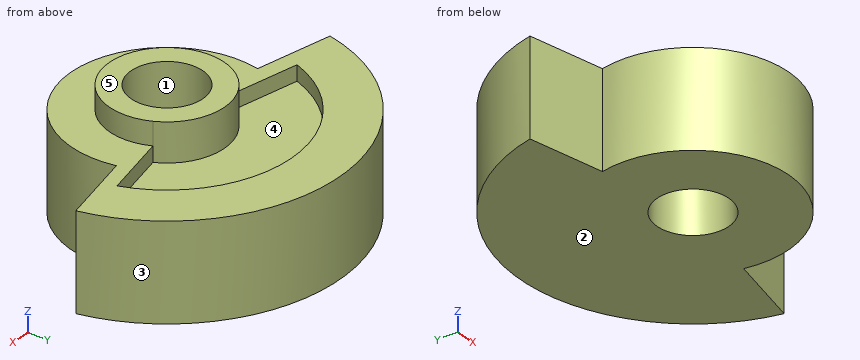
from build123d import *

# Parameters (mm, degrees)
SKETCH1_R           = 5
BOSS_EXTRUDE3_DEPTH = 6.2
SKETCH3_2_R         = 1.875
CUT_EXTRUDE2_DEPTH  = 10
CUT_EXTRUDE3_DEPTH  = 2
SKETCH5_R           = 10.344131343
SKETCH5_R_2         = 3
CUT_EXTRUDE4_DEPTH  = 1.2
SKETCH3_R           = 1.875
CUT_EXTRUDE1_DEPTH  = 5


with BuildPart() as part:
    # Sketch1 → Boss-Extrude3 (new body)
    with BuildSketch(Plane.XY):
        with BuildLine():
            ThreePointArc((-4.890844999, 1.039054952), (0, 5), (4.890844999, 1.039054952))
            Line((4.890844999, 1.039054952), (8.803520999, 1.870298914))
            ThreePointArc((8.803520999, 1.870298914), (0, 9), (-8.803520999, 1.870298914))
            Line((-8.803520999, 1.870298914), (-4.890844999, 1.039054952))
        make_face()
        Circle(SKETCH1_R)
    extrude(amount=BOSS_EXTRUDE3_DEPTH)

    # Sketch3_2 → Cut-Extrude2 (cut)
    with BuildSketch(Plane.XY.offset(6.2)):
        Circle(SKETCH3_2_R)
    extrude(amount=-CUT_EXTRUDE2_DEPTH, mode=Mode.SUBTRACT)

    # Sketch4 → Cut-Extrude3 (cut)
    with BuildSketch(Plane.XY.offset(6.2)):
        with BuildLine():
            Line((2.704066688, 1.299239525), (6.172842293, 2.036177308))
            ThreePointArc((6.172842293, 2.036177308), (0.066834303, 6.499656389), (-6.129666509, 2.162680856))
            Line((-6.129666509, 2.162680856), (-2.641748736, 1.42167634))
            ThreePointArc((-2.641748736, 1.42167634), (0.068691886, 2.999213468), (2.704066688, 1.299239525))
        make_face()
    extrude(amount=-CUT_EXTRUDE3_DEPTH, mode=Mode.SUBTRACT)

    # Sketch5 → Cut-Extrude4 (cut)
    with BuildSketch(Plane.XY.offset(6.2)):
        Circle(SKETCH5_R)
        Circle(SKETCH5_R_2, mode=Mode.SUBTRACT)
    extrude(amount=-CUT_EXTRUDE4_DEPTH, mode=Mode.SUBTRACT)

    # Sketch3 → Cut-Extrude1 (cut)
    with BuildSketch(Plane.XY.offset(6.2)):
        Circle(SKETCH3_R)
    extrude(amount=-CUT_EXTRUDE1_DEPTH, mode=Mode.SUBTRACT)


solid = part.part
The listing builds one solid part. Answer for the finished solid, in the listing's coordinates (mm). Face numbers are marked on the shaded views. A direction names the side the tool comes from. Coordinates: 2 decimals unless noted, no trailing zeros. Write each loop counter-clockwise with the first axis right and the second up, starting at its lowest first coordinate (ties: lowest second). Pieces come first, ordered by that corner, then holes. Notation, with made-up numbers: M 10.5,89 L 19.5,89 A19 ccw 19.5,119 Z; hole C 24.25,24.25 d1. An arc over 180 degrees is marked long. Put each result on its own line as item: value. Start each with the question number.
1. Consider line 1 (Y direction, x = 0, z = 4.5) (3 decimals); line 2 (Y direction, x = 0, z = 2) (3 decimals); line 3 (Z direction, x = -3.75, y = 3). Determine where each line is inside the solid, lowest interval first. Write a range as from..to.
2. A cutting plane is placed at D-D on x = 4. Write down the section's boundary in (y, z), then the cut area to 3 significant figures.
3. Which of the six approach directions +Z, -Z, +X, -X, +Y, -Y give full straight-line access (tool end or side, diameter ignored) to the marked faces 4 and 5?
4. A cutting plane is placed at A-A on y = 0. Write down the section's boundary in (x, z) (3 decimals).
5. A cutting plane is placed at C-C on z = 3.5. Write down the section's boundary in (x, y) (3 decimals), then the cut area to 3 significant figures.
6. Flat-ended cylindrical pins translate along their axes: P1, Ø1.5, axis at x = -5, y = 1.5, coming from the +Z side; P2, Ø1.6, axis at x = 2.5, y = 3.5, coming from the +Z side. Find the tip coordinate at first contact, or state that the pin passes through.
7. For a pull along Y with two mould halves and no side action, classify the marked faces 1, 2 and 3 as pulls with the +Y half, pulls with the -Y half, needs draft (parallel to the pull), parting line crosses it, or undercut.
8. A cutting plane is placed at B-B on x = 0. Write down the section's boundary in (y, z) (3 decimals), then the cut area to 4 significant figures.
Resolved:
1. line 1: y = -5..-1.875, 1.875..3, 6.5..9
1. line 2: y = -5..-1.875, 1.875..9
1. line 3: z = 0..4.2
2. outline: M -3,0 L 8.06,0 L 8.06,5 L 5.12,5 L 5.12,4.2 L 1.57,4.2 L 1.57,5 L -3,5 Z
2. area: 52.5 mm2
3. face 4: +Z
3. face 5: +Z, +X, -X, +Y, -Y
4. outline: M -5,0 L -1.875,0 L -1.875,6.2 L -3,6.2 L -3,5 L -5,5 Z; M 1.875,0 L 5,0 L 5,5 L 3,5 L 3,6.2 L 1.875,6.2 Z
5. outline: M -8.804,1.87 L -4.891,1.039 A5 ccw long 4.891,1.039 L 8.804,1.87 A9 ccw Z; hole C 0,0 d3.75
5. area: 144 mm2
6. P1: stops at z = 5
6. P2: stops at z = 4.2
7. face 1: undercut
7. face 2: needs draft
7. face 3: pulls with the +Y half
8. outline: M -5,0 L -1.875,0 L -1.875,6.2 L -3,6.2 L -3,5 L -5,5 Z; M 1.875,0 L 9,0 L 9,5 L 6.5,5 L 6.5,4.2 L 3,4.2 L 3,6.2 L 1.875,6.2 Z
8. area: 51.15 mm2
